from build123d import *

# Parameters (mm, degrees)
SKETCH1_W           = 25.4
SKETCH1_H           = 12.7
BOSS_EXTRUDE1_DEPTH = 12.7
FILLET1_R           = 3.175
SKETCH2_R           = 2.75
CUT_EXTRUDE1_DEPTH  = 32.108519733
BOSS_EXTRUDE2_START = 1.27
SKETCH3_W           = 27.94
SKETCH3_H           = 15.24
SKETCH3_R           = 2.75
BOSS_EXTRUDE2_DEPTH = 1.27
FILLET2_R           = 3.175


with BuildPart() as part:
    # Sketch1 → Boss-Extrude1 (new body)
    with BuildSketch(Plane(origin=(0, 0, 0), x_dir=(1, 0, 0), z_dir=(0, 1, 0))):
        with Locations((12.7, 6.35)):
            Rectangle(SKETCH1_W, SKETCH1_H)
    extrude(amount=BOSS_EXTRUDE1_DEPTH)

    # Fillet1
    fillet1_edges = [part.edges().sort_by_distance(p)[0] for p in [
        (25.4, 6.35, -12.7),
        (25.4, 6.35, 0),
    ]]
    fillet(fillet1_edges, radius=FILLET1_R)

    # Sketch2 → Cut-Extrude1 (cut, through all)
    with BuildSketch(Plane(origin=(0, 12.7, 0), x_dir=(1, 0, 0), z_dir=(0, 1, 0))):
        with Locations(Location((10, 6.35, 0), (0, 0, 270))):
            Circle(SKETCH2_R)
    extrude(amount=-CUT_EXTRUDE1_DEPTH, mode=Mode.SUBTRACT)

    # Sketch3 → Boss-Extrude2 (add)
    with BuildSketch(Plane(origin=(0, 12.7, 0), x_dir=(1, 0, 0), z_dir=(0, 1, 0)).offset(BOSS_EXTRUDE2_START)):
        with Locations((12.7, 6.35)):
            Rectangle(SKETCH3_W, SKETCH3_H)
        with Locations(Location((10, 6.35, 0), (0, 0, 270))):
            Circle(SKETCH3_R, mode=Mode.SUBTRACT)
    extrude(amount=-BOSS_EXTRUDE2_DEPTH)

    # Fillet2
    fillet2_edges = [part.edges().sort_by_distance(p)[0] for p in [
        (-1.27, 13.335, -13.97),
        (-1.27, 13.335, 1.27),
        (26.67, 13.335, 1.27),
        (26.67, 13.335, -13.97),
    ]]
    fillet(fillet2_edges, radius=FILLET2_R)


solid = part.part
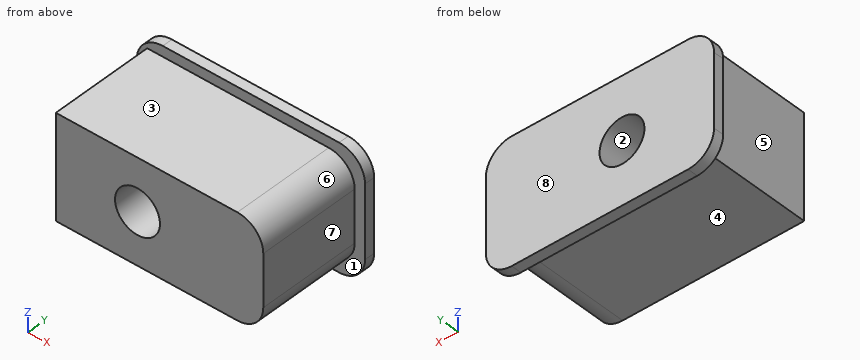
Geometry check sheet. Reference: the model listing, model coordinates, mm. Face numbers are marked on the shaded views. A direction names the side the tool comes from. Round coordinates to 2 decimals unless told otherwise and drop trailing zeros. Order: outer loops, then holes, each group sorted by start corner. A loop starts at its lowest first (then second) coordinate and runs counter-clockwise, first axis right, second up. Notation, with made-up numbers: (-32, 39.25) -> (5, 39.25) arc R18 cw to (5, 53.25) -> close; hole circle Ø4 at (-24.5, 4). An arc over 180 degrees is marked (long way). Use one line per item in the form item = value.
1. Go/stop test with flat-tipped pins: pin 1 (1.5 mm diameter, centred on x = 6, y = 3, fed in from -Z); pin 2 (4 mm diameter, centred on x = 14, y = 8, fed in from +Z); pin 3 (2 mm diameter, centred on y = 4.5, z = -12, fed in from -X). Record where each tip stops, or that it passes through.
Working result:
pin_1 = -12.7
pin_2 = 0
pin_3 = 0
2. Mould release check, pull along Z, two halves, no side actions. Record for the marked faces 1, 2, 3 and 4: pulls with the +Z half, pulls with the -Z half, needs draft (parallel to the pull), parting line crosses it, or undercut.
Working result:
face_1 = needs draft
face_2 = undercut
face_3 = pulls with the +Z half
face_4 = pulls with the -Z half
3. Set-up check for the marked faces 5, 6, 7 and 8: record each of +Z, -Z, +X, -X, +Y, -Y from which the full face is reachable in a straight line by a thin tool's end or side.
Working result:
face_5 = +Z, -Z, -X, -Y
face_6 = +Z, +X, -Y
face_7 = +Z, -Z, +X, -Y
face_8 = +Z, -Z, +X, -X, +Y
4. Scan lines: line 1 along X through (y, z) = (10, -6.35); line 2 along Z through (x, y) = (21.5, 4); line 3 along Z through (x, y) = (10.5, 4). Record each from-to range of solid material in increasing order. Write a range as from..to.
Working result:
line_1 = 0..7.25, 12.75..25.4
line_2 = -12.7..0
line_3 = -12.7..-9.05, -3.65..0
5. Cross-section at A-A, the plane x = 10. Enter the section's corners in (y, z).
Working result:
outline = (0, -12.7) -> (12.7, -12.7) -> (12.7, -13.97) -> (13.97, -13.97) -> (13.97, -9.1) -> (0, -9.1) -> close; (0, -3.6) -> (13.97, -3.6) -> (13.97, 1.27) -> (12.7, 1.27) -> (12.7, 0) -> (0, 0) -> close
6. Cross-section at B-B, the plane z = -6.35. Enter the section's corners in (x, y), plus the area to 3 significant figures.
Working result:
outline = (-1.27, 12.7) -> (0, 12.7) -> (0, 0) -> (7.25, 0) -> (7.25, 13.97) -> (-1.27, 13.97) -> close; (12.75, 0) -> (25.4, 0) -> (25.4, 12.7) -> (26.67, 12.7) -> (26.67, 13.97) -> (12.75, 13.97) -> close
area = 281 mm^2
7. Cross-section at C-C, the plane y = 8. Enter the section's corners in (x, z) (3 decimals).
Working result:
outline = (0, -12.7) -> (22.225, -12.7) arc R3.175 ccw to (25.4, -9.525) -> (25.4, -3.175) arc R3.175 ccw to (22.225, 0) -> (0, 0) -> close; hole circle Ø5.5 at (10, -6.35)
8. Cross-section at D-D, the plane x = 6.5. Enter the section's corners in (y, z).
Working result:
outline = (0, -12.7) -> (12.7, -12.7) -> (12.7, -13.97) -> (13.97, -13.97) -> (13.97, 1.27) -> (12.7, 1.27) -> (12.7, 0) -> (0, 0) -> close
